The listing builds one solid part. Answer for the finished solid, in the listing's coordinates (mm). Coordinates: 2 decimals unless noted, no trailing zeros. Loops run counter-clockwise (first coordinate to the right, second up) from the corner with the lowest first, then second, coordinate; pieces in that order, holes last. Notation, with made-up numbers: M -6.75,-31 L 44.25,-31 A17 cw 44.25,-13 Z; hole C -9,53.5 d1. An arc over 180 degrees is marked long. Return JSON: item names as keys, results as strings. Group by question number.
1. Section D-D (y = -3.75) is taken. Write down the section's boundary in (x, z), then the cut area to 3 significant figures.
2. Section A-A (x = 0) is taken. Write down the section's boundary in (y, z) (3 decimals).
3. Given P1, Ø3, axis at x = 2.5, z = -1.5, coming from the +Y side; P2, Ø3, axis at y = -4, z = -1, coming from the +X side; P3, Ø4, axis at y = -7.5, z = -6, coming from the -X side, each flat-ended and moving along its own axis, determine where each tip first touches the part or whether it passes through.
4. Section C-C (z = -2) is taken. Write down the section's boundary in (x, y).
5. Straight lines are drawn through the part: L1, parallel to Y at x = 5.75, z = -4; L2, parallel to X at y = -3, z = -3; L3, parallel to X at y = -5.5, z = -2.75. For each, find the intervals that lie inside material, in ascending order. Write a range as from..to.
6. Section B-B (z = -0.75) is taken. Write down the section's boundary in (x, y).
7. The mould has two halves that part along Z. Classify faces 1 (the face through (0, 0, -0.1)), 2 (the face through (0, 0, -5.9)), 3 (the face through (6.394, -4.419, -2.958)): pulls with the +Z half, pulls with the -Z half, needs draft (parallel to the pull), parting line crosses it, or undercut.
```python
from build123d import *

# Parameters (mm, degrees)
SKETCH1_R           = 0.5
BOSS_EXTRUDE1_DEPTH = 1
SKETCH2_R           = 0.45
CUT_EXTRUDE1_DEPTH  = 0.9
SKETCH3_R           = 0.225
BOSS_EXTRUDE2_DEPTH = 0.7
BOSS_EXTRUDE3_DEPTH = 6


with BuildPart() as part:
    # Sketch1 → Boss-Extrude1 (new body)
    with BuildSketch(Plane.XY):
        Circle(SKETCH1_R)
    boss_extrude1 = extrude(amount=-BOSS_EXTRUDE1_DEPTH)

    # Sketch2 → Cut-Extrude1 (cut)
    with BuildSketch(Plane(origin=(0, 0, -1), x_dir=(-1, 0, 0), z_dir=(0, 0, -1))):
        Circle(SKETCH2_R)
    cut_extrude1 = extrude(amount=-CUT_EXTRUDE1_DEPTH, mode=Mode.SUBTRACT)

    # Sketch3 → Boss-Extrude2 (add)
    with BuildSketch(Plane.XY):
        Circle(SKETCH3_R)
    boss_extrude2 = extrude(amount=BOSS_EXTRUDE2_DEPTH)

    # Sketch4 → Boss-Extrude3 (add)
    with BuildSketch(Plane.XY):
        with BuildLine():
            Line((12.615455291, -8.546775908), (0.5, 0))
            ThreePointArc((0.5, 0), (0.461939766, -0.191341716), (0.353553391, -0.353553391))
            Line((0.353553391, -0.353553391), (12.606131889, -8.600771882))
            Line((12.606131889, -8.600771882), (13.464797628, -8.38108067))
            Line((13.464797628, -8.38108067), (13.452404243, -8.332640975))
            Line((13.452404243, -8.332640975), (12.615455291, -8.546775908))
        make_face()
    extrude(amount=-BOSS_EXTRUDE3_DEPTH)

    # Mirror1: Boss-Extrude1, Cut-Extrude1, Boss-Extrude2 across plane
    add(boss_extrude1.mirror(Plane.XY.offset(-3)))
    add(cut_extrude1.mirror(Plane.XY.offset(-3)), mode=Mode.SUBTRACT)
    add(boss_extrude2.mirror(Plane.XY.offset(-3)))


solid = part.part
```
Worked out:
{
 "1": {"outline": "M 5.4,-6 L 5.82,-6 L 5.82,0 L 5.4,0 Z", "area": "2.50 mm^2"},
 "2": {"outline": "M -0.5,-6 L -0.225,-6 L -0.225,-6.7 L 0.225,-6.7 L 0.225,-6 L 0.5,-6 L 0.5,-5 L 0.45,-5 L 0.45,-5.9 L -0.45,-5.9 L -0.45,-5 L -0.5,-5 Z; M -0.5,-1 L -0.45,-1 L -0.45,-0.1 L 0.45,-0.1 L 0.45,-1 L 0.5,-1 L 0.5,0 L 0.225,0 L 0.225,0.7 L -0.225,0.7 L -0.225,0 L -0.5,0 Z"},
 "3": {"P1": "y = -0.35", "P2": "x = 8.3", "P3": "x = 8"},
 "4": {"outline": "M 0.35,-0.35 L 12.61,-8.6 L 13.46,-8.38 L 13.45,-8.33 L 12.62,-8.55 L 0.5,0 A0.5 cw Z"},
 "5": {"L1": "-3.99..-3.7", "L2": "4.29..4.75", "L3": "8..8.3"},
 "6": {"outline": "M 0.35,-0.35 L 12.61,-8.6 L 13.46,-8.38 L 13.45,-8.33 L 12.62,-8.55 L 0.5,0 A0.5 ccw long Z; hole C 0,0 d0.9"},
 "7": {"face 1": "undercut", "face 2": "undercut", "face 3": "needs draft"}
}
